Input: part model. Units: mm. Frame: model coordinates. Give positions to 0.01 mm unless a question says otherwise; leave off trailing zeros. Use CSV: the item, a comma, the result in double quotes. Start each with the question number.
from build123d import *

# Parameters (mm, degrees)
BOSS_EXTRUDE1_DEPTH     = 300
SKETCH3_R               = 15.5
CUT_EXTRUDE1_DEPTH      = 23
CUT_EXTRUDE1_DEPTH_BACK = 23
SKETCH4_R               = 35
CUT_EXTRUDE3_DEPTH      = 300
SKETCH5_W               = 496.22566609
SKETCH5_H               = 70.680473068
SKETCH5_W_2             = 504.512342242
SKETCH5_H_2             = 238.363802277
CUT_EXTRUDE4_DEPTH      = 201.0000001


with BuildPart() as part:
    # Sketch1 → Boss-Extrude1 (new body)
    with BuildSketch(Plane(origin=(0, 0, 0), x_dir=(1, 0, 0), z_dir=(0, 1, 0))):
        with BuildLine():
            Line((-200, 1e-09), (200, 1e-09))
            add(Edge.make_bspline(
                [(-200, 1e-09), (0, -400.000000001), (200, 1e-09)],
                knots=[0.056028396, 0.056028396, 0.056028396, 0.943971604, 0.943971604, 0.943971604], degree=2))
        make_face()
    extrude(amount=BOSS_EXTRUDE1_DEPTH)

    # Sketch3 → Cut-Extrude1 (cut, two sides)
    with BuildSketch(Plane(origin=(0, 150, 0), x_dir=(1, 0, 0), z_dir=(0, 1, 0))) as cut_extrude1_sk:
        with Locations((0, -142.999999999)):
            Circle(SKETCH3_R)
    extrude(amount=CUT_EXTRUDE1_DEPTH, mode=Mode.SUBTRACT)
    extrude(cut_extrude1_sk.sketch, amount=-CUT_EXTRUDE1_DEPTH_BACK, mode=Mode.SUBTRACT)

    # Sketch4 → Cut-Extrude3 (cut)
    with BuildSketch(Plane(origin=(0, 173, 0), x_dir=(1, 0, 0), z_dir=(0, 1, 0))):
        with Locations((0, -142.999999999)):
            Circle(SKETCH4_R)
    cut_extrude3 = extrude(amount=CUT_EXTRUDE3_DEPTH, mode=Mode.SUBTRACT)

    # Mirror1: Cut-Extrude3 across plane
    add(cut_extrude3.mirror(Plane.ZX.offset(150)), mode=Mode.SUBTRACT)

    # Sketch5 → Cut-Extrude4 (cut, through all)
    with BuildSketch(Plane(origin=(0, 0, 0), x_dir=(-1, 0, 0), z_dir=(0, 0, -1))):
        with Locations((-4.143338076, 284.540236534)):
            Rectangle(SKETCH5_W, SKETCH5_H)
        with Locations((0, 79.218098862)):
            Rectangle(SKETCH5_W_2, SKETCH5_H_2)
    extrude(amount=-CUT_EXTRUDE4_DEPTH, mode=Mode.SUBTRACT)


solid = part.part
Item 1: First-contact query: pin 1 Ø12 at (x, y) = (67, 224.5) entering from +Z (3 decimals); pin 2 Ø8 at (y, z) = (229.5, 167.5) entering from -X; pin 3 Ø2 at (y, z) = (209.5, 175) entering from +X. Flat tips, straight axial feed; report the tip coordinate or a pass-through.
Item 2: Material intervals for line 1 (Z direction, x = 0, y = 219); line 2 (X direction, y = 231, z = 148); line 3 (X direction, y = 204, z = 164.5), sorted ascending.
Item 3: Mould query, pull axis Z, two halves, no side actions, for faces 1 (the flat face through (-3, 223, 0)), 2 (the cylindrical face through (-7.587, 223.444, 177.168)), 3 (the flat face through (3, 198.4, 76)). Classes: +Z half, -Z half, draft (parallel to the pull), parting line (faces both ways), or undercut.
Recorded:
1,pin 1,"z = 181.395"
1,pin 2,"x = -85.44"
1,pin 3,"x = 72.11"
2,line 1,"0 to 108, 178 to 200"
2,line 2,"-101.98 to -34.64, 34.64 to 101.98"
2,line 3,"-84.26 to -27.62, 27.62 to 84.26"
3,face 1,"-Z half"
3,face 2,"undercut"
3,face 3,"draft"
